Read the model definition and answer for the solid it produces. Units are mm, in the model's axes. A direction names the side the tool comes from. Coordinates: 2 decimals unless noted, no trailing zeros. Order: outer loops, then holes, each group sorted by start corner. A loop starts at its lowest first (then second) coordinate and runs counter-clockwise, first axis right, second up. Notation, with made-up numbers: M 68.5,-34.75 L 118.5,-34.75 A8 cw 118.5,-23.75 Z; hole C 27.25,71 d1. An arc over 180 degrees is marked long. Use a Markdown table: item, result. Add a question column.
1) For faces 1 (the face through (0, 0, 0)), 2 (the face through (13.18, 68.465, 9.645)), 3 (the face through (-9.645, 68.465, 13.18)), 4 (the face through (-11, 71, 4)), determine the directions among +Z, -Z, +X, -X, +Y, -Y from which every point of the face is accessible in a straight line to the end or side of a thin tool.
2) Each of these flat-tipped pins is pushed along its axis until it touches: pin 1 Ø5 at (x, y) = (11.5, 22.5) entering from -Z; pin 2 Ø2 at (x, z) = (12.5, -11.5) entering from +Y; pin 3 Ø3 at (y, z) = (44, -6) entering from -X. Where does it stop, or does it pass through?
3) The mould has two halves that part along Z. Classify faces 5 (the face through (-10.648, 16.297, -13.887)), 6 (the face through (14.45, 68.54, 1.43)), 7 (the face through (0.07, 68.54, 12.5)), 8 (the face through (-13.213, 68.465, -9.677)): released by +Z, released by -Z, zero draft, split by the parting line, or undercut.
4) Find section C-C on y = 34. Write down the section's boundary in (x, z), plus the area to 3 significant figures.
5) Find section A-A on z = 0. Write down the section's boundary in (x, y), plus the area to 3 significant figures.
6) Find section B-B on y = 6. Write down the section's boundary in (x, z).
7) Find the intervals of material crossed by probe 1 along X at (y, z) = (67, 0); probe 2 along X at (y, z) = (67.5, -9.5); probe 3 along X at (y, z) = (72.15, 0), in increasing order. Write a range as [from, to].
from build123d import *

# Parameters (mm, degrees)
SKETCH1_R           = 17.5
BOSS_EXTRUDE1_DEPTH = 31
SKETCH2_R           = 18
BOSS_EXTRUDE2_DEPTH = 40
FILLET1_R           = 2
FILLET2_R           = 1
SKETCH3_R           = 11
BOSS_EXTRUDE3_DEPTH = 2.3
SKETCH4_R           = 4
CUT_EXTRUDE1_DEPTH  = 3
SKETCH5_R           = 1.5
CUT_EXTRUDE2_DEPTH  = 5
FILLET3_R           = 1
CUT_EXTRUDE3_START  = -5
CUT_EXTRUDE3_DEPTH  = 5


with BuildPart() as part:
    # Sketch1 → Boss-Extrude1 (new body)
    with BuildSketch(Plane(origin=(0, 0, 0), x_dir=(1, 0, 0), z_dir=(0, 1, 0))):
        with Locations(Location((0, 0, 0), (0, 0, 270))):
            Circle(SKETCH1_R)
    extrude(amount=BOSS_EXTRUDE1_DEPTH)

    # Sketch2 → Boss-Extrude2 (add)
    with BuildSketch(Plane(origin=(0, 31, 0), x_dir=(1, 0, 0), z_dir=(0, 1, 0))):
        with Locations(Location((0, 0, 0), (0, 0, 270))):
            Circle(SKETCH2_R)
    extrude(amount=BOSS_EXTRUDE2_DEPTH)

    # Fillet1
    fillet1_edges = [part.edges().sort_by_distance(p)[0] for p in [
        (0, 0, -17.5),
    ]]
    fillet(fillet1_edges, radius=FILLET1_R)

    # Fillet2
    # the kernel refuses this fillet: 1 mm, written as the material it takes off along each edge
    with BuildSketch(Plane(origin=(0, 31, 0), x_dir=(0, 0, 1), z_dir=(-1, 0, 0))) as fillet2_piece_1:
        with BuildLine():
            CenterArc((17, 0.866025404), FILLET2_R, 300, 60)
            Line((18, 0.866025404), (18.02, 0.866025404))
            Line((18.02, 0.866025404), (18.02, 0))
            Line((18.02, 0), (18, -0.02))
            ThreePointArc((18, -0.02), (17.75, -0.02), (17.51, -0.017320508))
            Line((17.51, -0.017320508), (17.5, 0))
        make_face()
    revolve(axis=Axis((0, 31, 0), (0, 1, 0)), mode=Mode.SUBTRACT)

    # Sketch3 → Boss-Extrude3 (add)
    with BuildSketch(Plane(origin=(0, 71, 0), x_dir=(1, 0, 0), z_dir=(0, 1, 0))):
        with Locations(Location((0, 0, 0), (0, 0, 270))):
            Circle(SKETCH3_R)
    extrude(amount=BOSS_EXTRUDE3_DEPTH)

    # Sketch4 → Cut-Extrude1 (cut)
    with BuildSketch(Plane(origin=(0, 73.3, 0), x_dir=(1, 0, 0), z_dir=(0, 1, 0))):
        with Locations(Location((0, 0, 0), (0, 0, 270))):
            Circle(SKETCH4_R)
    extrude(amount=-CUT_EXTRUDE1_DEPTH, mode=Mode.SUBTRACT)

    # Sketch5 → Cut-Extrude2 (cut)
    with BuildSketch(Plane(origin=(0, 71, 0), x_dir=(1, 0, 0), z_dir=(0, 1, 0))):
        with Locations(Location((-14, 0, 0), (0, 0, 270))):
            Circle(SKETCH5_R)
        with Locations(Location((0, 14, 0), (0, 0, 270))):
            Circle(SKETCH5_R)
        with Locations(Location((14, 0, 0), (0, 0, 270))):
            Circle(SKETCH5_R)
        with Locations(Location((0, -14, 0), (0, 0, 270))):
            Circle(SKETCH5_R)
    extrude(amount=-CUT_EXTRUDE2_DEPTH, mode=Mode.SUBTRACT)

    # Fillet3
    fillet3_edges = [part.edges().sort_by_distance(p)[0] for p in [
        (0, 71, -18),
    ]]
    fillet(fillet3_edges, radius=FILLET3_R)

    # Sketch6 → Cut-Extrude3 (cut)
    with BuildSketch(Plane(origin=(0, 71, 0), x_dir=(1, 0, 0), z_dir=(0, 1, 0)).offset(CUT_EXTRUDE3_START)):
        with BuildLine():
            Line((-14.372329619, 10.836795713), (-12.02081528, 8.485281374))
            ThreePointArc((-12.02081528, 8.485281374), (-8.485281374, 8.485281374), (-8.485281374, 12.02081528))
            Line((-8.485281374, 12.02081528), (-10.836795713, 14.372329619))
            ThreePointArc((-10.836795713, 14.372329619), (-12.727922061, 12.727922061), (-14.372329619, 10.836795713))
        make_face()
        with BuildLine():
            Line((14.372329619, 10.836795713), (12.02081528, 8.485281374))
            ThreePointArc((12.02081528, 8.485281374), (8.485281374, 8.485281374), (8.485281374, 12.02081528))
            Line((8.485281374, 12.02081528), (10.836795713, 14.372329619))
            ThreePointArc((10.836795713, 14.372329619), (12.727922061, 12.727922061), (14.372329619, 10.836795713))
        make_face()
        with BuildLine():
            Line((10.836795713, -14.372329619), (8.485281374, -12.02081528))
            ThreePointArc((8.485281374, -12.02081528), (8.485281374, -8.485281374), (12.02081528, -8.485281374))
            Line((12.02081528, -8.485281374), (14.372329619, -10.836795713))
            ThreePointArc((14.372329619, -10.836795713), (12.727922061, -12.727922061), (10.836795713, -14.372329619))
        make_face()
        with BuildLine():
            Line((-14.372329619, -10.836795713), (-12.02081528, -8.485281374))
            ThreePointArc((-12.02081528, -8.485281374), (-8.485281374, -8.485281374), (-8.485281374, -12.02081528))
            Line((-8.485281374, -12.02081528), (-10.836795713, -14.372329619))
            ThreePointArc((-10.836795713, -14.372329619), (-12.727922061, -12.727922061), (-14.372329619, -10.836795713))
        make_face()
    extrude(amount=CUT_EXTRUDE3_DEPTH, mode=Mode.SUBTRACT)


solid = part.part
Check result:
| question | item | result |
|---|---|---|
| 1 | face 1 | +Z, -Z, +X, -X, -Y |
| 1 | face 2 | +Z, +Y |
| 1 | face 3 | -X, +Y |
| 1 | face 4 | +Y |
| 2 | pin 1 | stops at z = -15.01 |
| 2 | pin 2 | stops at y = 66 |
| 2 | pin 3 | stops at x = -17.43 |
| 3 | face 5 | split by the parting line |
| 3 | face 6 | undercut |
| 3 | face 7 | undercut |
| 3 | face 8 | released by -Z |
| 4 | outline | C 0,0 d36 |
| 4 | area | 1,020 mm2 |
| 5 | outline | M -18,31.87 A1 ccw -17.5,31 L -17.5,2 A2 ccw -15.5,0 L 15.5,0 A2 ccw 17.5,2 L 17.5,31 A1 ccw 18,31.87 L 18,70 A1 ccw 17,71 L 15.5,71 L 15.5,66 L 12.5,66 L 12.5,71 L 11,71 L 11,73.3 L 4,73.3 L 4,70.3 L -4,70.3 L -4,73.3 L -11,73.3 L -11,71 L -12.5,71 L -12.5,66 L -15.5,66 L -15.5,71 L -17,71 A1 ccw -18,70 Z |
| 5 | area | 2,520 mm2 |
| 6 | outline | C 0,0 d35 |
| 7 | probe 1 | x = [-18, -15.5], [-12.5, 12.5], [15.5, 18] |
| 7 | probe 2 | x = [-15.29, -13.04], [-7.87, 7.87], [13.04, 15.29] |
| 7 | probe 3 | x = [-11, -4], [4, 11] |
